Read the model definition and answer for the solid it produces. Units are mm, in the model's axes. A direction names the side the tool comes from. Coordinates: 2 decimals unless noted, no trailing zeros. Write each loop counter-clockwise with the first axis right and the second up, starting at its lowest first coordinate (ties: lowest second). Pieces come first, ordered by that corner, then holes. Notation, with made-up numbers: (73.5, 41) -> (98.5, 41) arc R20 cw to (98.5, 80) -> close; hole circle Ø1 at (32, 47.25). An arc over 180 degrees is marked (long way). Answer as a JSON object with one key per item and string values. Group by question number.
(1) For a pull along Y with two mould halves and no side action, classify faces 3 (the face through (0.338, 2.578, 6.58)), 4 (the face through (-7, 0, 4)), 5 (the face through (3, -3, 0)) as +Y half, -Y half, draft (parallel to the pull), parting line (faces both ways), or undercut.
(2) Which of the six approach directions +Z, -Z, +X, -X, +Y, -Y give full straight-line access (tool end or side, diameter ignored) to faces 1 (the face through (-1, -3, 5.2)), 2 (the face through (6.499, 0, 4))?
(3) Flat-ended cylindrical pins translate along their axes: P1, Ø2, axis at x = -2, z = 2, coming from the -Y side; P2, Ø3, axis at x = 0, y = 0, coming from the +Z side; P3, Ø1.5, axis at x = 2, z = 1, coming from the +Y side; P4, Ø1, axis at x = -3, z = 5, coming from the +Y side. Find the tip coordinate at first contact, or state that the pin passes through.
(4) Find section A-A (x = 0). Give the vertices of the cut face in (y, z), then the cut area to 3 significant figures.
(5) Find section D-D (z = 5.5). Give the vertices of the cut face in (x, y), then the cut area to 3 significant figures.
(6) Find section C-C (y = 3). Give the vertices of the cut face in (x, z).
(7) Straight lines are drawn through the part: L1, parallel to Y at x = 0, z = 6.4; L2, parallel to Y at x = 0, z = 1.75; L3, parallel to X at y = -2.5, z = 3. For each, find the intervals that lie inside material, in ascending order.
(8) Find section B-B (y = 0). Give the vertices of the cut face in (x, z).
from build123d import *

# Parameters (mm, degrees)
EXTRUDE_1_DEPTH     = 8
SKETCH_2_R          = 3.95
CUT_EXTRUDE_1_DEPTH = 5.2
SKETCH_3_R          = 2.6
CUT_EXTRUDE_2_DEPTH = 5.2


with BuildPart() as part:
    # Эскиз1 → Бобышка-Вытянуть1 (new body)
    with BuildSketch(Plane.XY):
        with BuildLine():
            Line((6.498674865, -2.601389052), (6.498674865, 2.601389052))
            ThreePointArc((6.498674865, 2.601389052), (-7, 0), (6.498674865, -2.601389052))
        make_face()
    extrude(amount=EXTRUDE_1_DEPTH)

    # Эскиз2 → Вырез-Вытянуть1 (cut)
    with BuildSketch(Plane(origin=(0, 0, 0), x_dir=(-1, 0, 0), z_dir=(0, 0, -1))):
        Circle(SKETCH_2_R)
    extrude(amount=-CUT_EXTRUDE_1_DEPTH, mode=Mode.SUBTRACT)

    # Эскиз3 → Вырез-Вытянуть2 (cut)
    with BuildSketch(Plane(origin=(0, 0, 5.2), x_dir=(-1, 0, 0), z_dir=(0, 0, -1))):
        Circle(SKETCH_3_R)
    extrude(amount=-CUT_EXTRUDE_2_DEPTH, mode=Mode.SUBTRACT)


solid = part.part
Results below:
{
 "1": {"face 3": "undercut", "face 4": "parting line", "face 5": "draft"},
 "2": {"face 1": "-Z", "face 2": "+Z, -Z, +X, +Y, -Y"},
 "3": {"P1": "stops at y = -6.93", "P2": "passes through", "P3": "stops at y = 6.89", "P4": "stops at y = 6.54"},
 "4": {"outline": "(-7, 0) -> (-3.95, 0) -> (-3.95, 5.2) -> (-2.6, 5.2) -> (-2.6, 8) -> (-7, 8) -> close; (2.6, 5.2) -> (3.95, 5.2) -> (3.95, 0) -> (7, 0) -> (7, 8) -> (2.6, 8) -> close", "area": "56.4 mm2"},
 "5": {"outline": "(6.5, -2.6) -> (6.5, 2.6) arc R7 ccw (long way) to start; hole circle Ø5.2 at (0, 0)", "area": "131 mm2"},
 "6": {"outline": "(-6.32, 0) -> (-2.57, 0) -> (-2.57, 5.2) -> (2.57, 5.2) -> (2.57, 0) -> (6.32, 0) -> (6.32, 8) -> (-6.32, 8) -> close"},
 "7": {"L1": "y = -7 to -2.6, 2.6 to 7", "L2": "y = -7 to -3.95, 3.95 to 7", "L3": "x = -6.54 to -3.06, 3.06 to 6.5"},
 "8": {"outline": "(-7, 0) -> (-3.95, 0) -> (-3.95, 5.2) -> (-2.6, 5.2) -> (-2.6, 8) -> (-7, 8) -> close; (2.6, 5.2) -> (3.95, 5.2) -> (3.95, 0) -> (6.5, 0) -> (6.5, 8) -> (2.6, 8) -> close"}
}
